Autodesk Inventor part; units mm, degrees
ref_plane "YZ Plane" through (0, 0, 0) normal (1, 0, 0) x (0, 1, 0)
ref_plane "XZ Plane" through (0, 0, 0) normal (0, 1, 0) x (-1, 0, 0)
ref_plane "XY Plane" through (0, 0, 0) normal (0, 0, 1) x (1, 0, 0)
sketch "Sketch1" plane through (0, 0, 0) normal (0, 1, 0) x (-1, 0, 0)
  line L0 (0, 0) -> (0, 10)
  line L1 (0, 10) -> (42.1132, 10)
  line L2 (0, 0) -> (36.3397, 0)
  line L3 (40.6699, -2.5) -> (86.3115, -81.5535)
  line L4 (86.9054, -84.9218) -> (86.0202, -89.942)
  line L5 (90.076, -95.7343) -> (90.076, -95.7343)
  line L6 (95.8682, -91.6785) -> (97.3855, -83.0739)
  line L7 (96.7916, -79.7056) -> (46.4434, 7.5)
  arc A0 (45.5774, 9) -> (43.8453, 10) centre (43.8453, 8) ccw
  arc A1 (40.6699, -2.5) -> (36.3397, 0) centre (36.3397, -5) ccw
  arc A2 (86.9054, -84.9218) -> (86.3115, -81.5535) centre (81.9813, -84.0535) ccw
  arc A3 (97.3855, -83.0739) -> (96.7916, -79.7056) centre (92.4614, -82.2056) ccw
  arc A4 (46.4434, 7.5) -> (42.1132, 10) centre (42.1132, 5) ccw
  arc A5 (90.076, -95.7343) -> (95.8682, -91.6785) centre (90.9442, -90.8103) ccw
  arc A6 (86.0202, -89.942) -> (90.076, -95.7343) centre (90.9442, -90.8103) ccw
  point P0 (85.1519, -94.8661)
  point P1 (95, -96.6025)
  point P2 (45, 10)
  point P3 (90.076, -95.7343)
  dimension "d1" = 120
  dimension "d2" = 140
  dimension "d3" = 45
  dimension "d4" = 50
  dimension "d5" = 10
  dimension "d6" = 10
  dimension "d7" = 10
  dimension "d8" = 2
  dimension "d9" = 5
extrude "Extrusion1" add sketch "Sketch1" along normal blind 3
sketch "Sketch2" plane through (0, 3, 0) normal (0, 1, 0) x (1, 0, 0)
  line L0 (0, -10) -> (0, 0)
  line L1 (0, -5) -> (-25.3234, -5) construction
  point P0 (-6.55, -5)
  dimension "d19" = 6.55
hole "Hole1" at (-6.55, 3, 5) direction (0, -1, 0) diameter 3.2 end through all
mirror "Mirror1" about plane through (0, 0, 0) normal (1, 0, 0) of "Extrusion1", "Hole1"
sketch "Sketch3" plane through (0, 3, 0) normal (0, 1, 0) x (1, 0, 0)
  line L0 (-40.6699, 2.5) -> (-86.3115, 81.5535)
  line L1 (-36.3397, 0) -> (36.3397, 0)
  arc A0 (-71.1338, 55.2651) -> (0, 0) centre (18.4247, 97.1272) ccw
  line L2 (-40.6699, 2.5) -> (-86.3115, 81.5535)
  arc A1 (-40.6699, 2.5) -> (-36.3397, 0) centre (-36.3397, 5) ccw
  point P0 (-62.6082, 40.4983)
extrude "Extrusion2" add sketch "Sketch3" against normal up to surface (3 mm away) contours L0 A0 L1 A1
mirror "Mirror2" about plane through (0, 0, 0) normal (1, 0, 0) of "Extrusion2"
fillet "Fillet1" radius 5 1 edges at (0, 1.5, 0)
sketch "Sketch4" plane through (0, 3, 0) normal (0, 1, 0) x (1, 0, 0)
  arc A0 (-62.6082, 40.4983) -> (-0.9815, 0.1913) centre (18.4247, 97.1272) ccw
  arc A1 (-70.805, 34.7701) -> (-2.9445, -9.6141) centre (18.4247, 97.1272) ccw
  line L0 (-96.7916, 79.7056) -> (-46.4434, -7.5)
  arc A2 (-46.4434, -7.5) -> (-42.1132, -10) centre (-42.1132, -5) ccw
  line L1 (-42.1132, -10) -> (42.1132, -10)
  line L2 (-16.55, -5.9607) -> (-16.55, -10)
  circle A3 centre (-6.55, -5) radius 1.6
  line L3 (-70.805, 34.7701) -> (-71.0577, 35.1332)
  point P0 (0, 0)
  point P1 (-16.55, -7.9804)
  dimension "d23" = 10
  dimension "d24" = 10
extrude "Extrusion3" cut sketch "Sketch4" against normal blind 10 contours A1 L2 L1 A2 L0 L3
fillet "Fillet2" radius 5 2 edges at (-16.55, 1.5, 5.9607) (-16.55, 1.5, 10)
mirror "Mirror3" about plane through (0, 0, 0) normal (1, 0, 0) of "Fillet2", "Extrusion3"
ref_plane "Work Plane1" through (-11.6432, 0, 0) normal (0, 0, 1) x (1, 0, 0)
sketch "Sketch5" plane through (-11.6432, 0, 0) normal (0, 0, 1) x (1, 0, 0)
  line L0 (0, 3) -> (23.2863, 3)
  line L1 (11.6432, 3) -> (11.6432, 0)
  line L2 (19.7932, 0) -> (16.5932, 0)
  line L3 (6.6932, 3) -> (16.5932, 3)
  line L4 (16.5932, 3) -> (16.5932, 0)
  line L5 (16.5932, 0) -> (6.6932, 0)
  line L6 (6.6932, 0) -> (6.6932, 3)
  line L7 (6.6932, 3) -> (16.5932, 0) construction
  line L8 (16.5932, 3) -> (6.6932, 0) construction
  point P0 (11.6432, 1.5)
extrude "Extrusion4" add sketch "Sketch5" against normal blind 1
fillet "Fillet3" radius 5 2 edges at (-4.6561, 1.5, -1) (4.6561, 1.5, -1)
properties part number "Claw1" material "Copper, Cast"
Input: part model. Units: mm. Frame: model coordinates. A direction names the side the tool comes from. Coordinates: 2 decimals unless noted, no trailing zeros. Loops run counter-clockwise (first coordinate to the right, second up) from the corner with the lowest first, then second, coordinate; pieces in that order, holes last. Notation, with made-up numbers: (46.25, -10.5) - (94.25, -10.5) arc R26 ccw to (94.25, 16.5) - close; hole circle Ø3 at (34, 58). An arc over 180 degrees is marked (long way). Answer in a Markdown table with one row per item. Add a question column.
Item 1: Section query C-C on x = 67.5. Return the cut outline in (y, z), then the cut area to 3 significant figures.
Item 2: Section query B-B on z = -68.5. Return the cut outline in (x, y), then the cut area to 3 significant figures.
Item 3: Section query D-D on x = 34. Return the cut outline in (y, z).
Item 4: Mould query, pull axis X, two halves, no side actions, for faces 1 (the cylindrical face through (-86.88, 1.48, -93.72)), 2 (the flat face through (0, 0, 0)), 3 (the flat face through (-84.105, 1.479, -57.731)). Classes: released by +X, released by -X, zero draft, split by the parting line, or undercut.
Item 5: Access query for faces 4 (the cylindrical face through (-37.916, 1.521, -15.894)), 5 (the cylindrical face through (47.443, 1.521, -10.457)). Directions: +Z, -Z, +X, -X, +Y, -Y. A direction counts if a zero-diameter tool reaches every point of the face in a straight line with its end or side. Return the directions, or none.
Item 6: Section query A-A on y = 1.3. State how many separate pieces and enclosed holes the cut face has, then the cut area to 3 significant figures.
Item 7: Contact query for flat-ended pins moving along their axis: P1, Ø3, axis at x = -6.55, z = 5, coming from the -Y side; P2, Ø1.5, axis at y = 1.5, z = -57, coming from the -X side. Output: stop coordinate, or through.
Item 8: Line query: line 1 along Z through (x, y) = (-6.55, 2.1); line 2 along X through (y, z) = (1.2, -34); line 3 along X through (y, z) = (2.2, -17.5). Output: solid intervals per line, ascending. Write a range as [from, to].
Recorded:
| question | item | result |
|---|---|---|
| 1 | outline | (0, -48.97) - (3, -48.97) - (3, -30.29) - (0, -30.29) - close |
| 1 | area | 56.0 mm^2 |
| 2 | outline | (-90.32, 0) - (-78.78, 0) - (-78.78, 3) - (-90.32, 3) - close; (78.78, 0) - (90.32, 0) - (90.32, 3) - (78.78, 3) - close |
| 2 | area | 69.3 mm^2 |
| 3 | outline | (0, -13.31) - (3, -13.31) - (3, -1.72) - (0, -1.72) - close |
| 4 | face 1 | undercut |
| 4 | face 2 | zero draft |
| 4 | face 3 | released by -X |
| 5 | face 4 | -Z, +Y, -Y |
| 5 | face 5 | +Z, +X, +Y, -Y |
| 6 | separate pieces | 1 |
| 6 | enclosed holes | 2 |
| 6 | area | 2,940 mm^2 |
| 7 | P1 | through |
| 7 | P2 | x = -84.12 |
| 8 | line 1 | [-1.47, 3.4], [6.6, 10] |
| 8 | line 2 | [-70.26, -57.65], [57.65, 70.26] |
| 8 | line 3 | [-55.8, -40.16], [40.16, 55.8] |
